from build123d import *

# Parameters (mm, degrees)
F0_R     = 3.048
F1_DEPTH = 6.35
F2_R     = 6.0325
F2_R_2   = 3.048
F3_DEPTH = 2.54
F5_DEPTH = 15.24
F6_R     = 1.397
F7_DEPTH = 9.525


with BuildPart() as f1:
    # F0 (on Top) → F1 (new body)
    with BuildSketch(Plane.XY):
        Circle(F0_R)
    extrude(amount=F1_DEPTH)

    # F2 (on face) → F3 (join)
    with BuildSketch(Plane(origin=(0, 0, 0), x_dir=(1, 0, 0), z_dir=(0, 0, -1))):
        Circle(F2_R)
        Circle(F2_R_2, mode=Mode.SUBTRACT)
        Circle(F2_R_2)
    extrude(amount=F3_DEPTH)

    # F4 (on face) → F5 (join)
    with BuildSketch(Plane(origin=(0, 0, -2.54), x_dir=(1, 0, 0), z_dir=(0, 0, -1))):
        Polygon((3.4925, -6.35), (-3.4925, 6.35), (-3.4925, -6.35), align=None)
        Polygon((3.4925, 6.35), (-3.4925, 6.35), (3.4925, -6.35), align=None)
    extrude(amount=F5_DEPTH)

    # F6 (on face) → F7 (join)
    with BuildSketch(Plane.XY.offset(6.35)):
        Circle(F6_R)
    extrude(amount=F7_DEPTH)


solid = f1.part
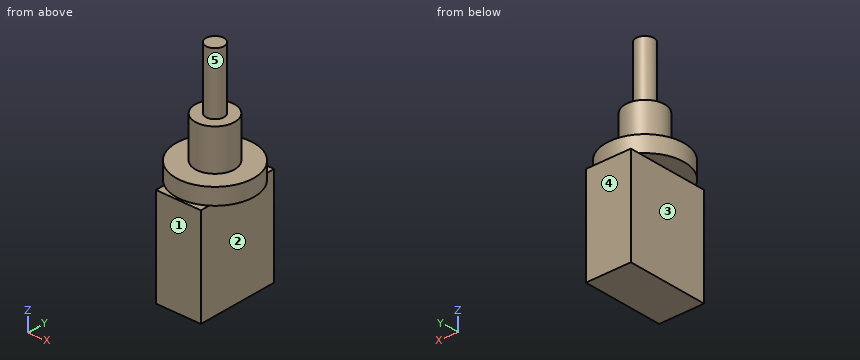
Geometry: final body of the model. Coordinates: model frame, mm. Face numbers are marked on the shaded views. A direction names the side the tool comes from. Round coordinates to 2 decimals unless told otherwise and drop trailing zeros. Loops run counter-clockwise (first coordinate to the right, second up) from the corner with the lowest first, then second, coordinate; pieces in that order, holes last. Notation, with made-up numbers: (-12.75, 27) - (-7.75, 27) arc R23 ccw to (-7.75, 56) - close; hole circle Ø11 at (31.5, -32). An arc over 180 degrees is marked (long way). Write each question's results on one line, items separated by ' | '. Start each with the question number.
1) Line query: probe 1 along X at (y, z) = (1.5, -12); probe 2 along Z at (x, y) = (0, 5.5); probe 3 along Z at (x, y) = (-1, 2.5). Output: solid intervals per line, ascending. Write a range as [from, to].
2) Cut plane C-C on z = 13.5. Return loops of the section in (x, y).
3) First-contact query: P1, Ø1.3, axis at x = 5.5, y = 0.5, coming from the -Z side; P2, Ø6, axis at x = -3, z = 9.5, coming from the +Y side; P3, Ø3, axis at x = 3.5, y = -2.5, coming from the +Z side. Flat tips, straight axial feed; report the tip coordinate or a pass-through.
4) Cut plane D-D on y = -3.75. Return loops of the section in (x, z).
5) Access query for the marked faces 1, 2, 3, 4 and 5. Directions: +Z, -Z, +X, -X, +Y, -Y. A direction counts if a zero-diameter tool reaches every point of the face in a straight line with its end or side. Return the directions, or none.
Verdict:
1) probe 1: x = [-3.49, 3.49] | probe 2: z = [-17.78, 0] | probe 3: z = [-17.78, 6.35]
2) outline: circle Ø2.79 at (0, 0)
3) P1: stops at z = -2.54 | P2: stops at y = 1.4 | P3: stops at z = 6.35
4) outline: (-4.73, -2.54) - (-3.49, -2.54) - (-3.49, -17.78) - (3.49, -17.78) - (3.49, -2.54) - (4.73, -2.54) - (4.73, 0) - (-4.73, 0) - close
5) face 1: +Z, -Z, +X, -X, -Y | face 2: -Z, +X, +Y, -Y | face 3: -Z, -X, +Y, -Y | face 4: +Z, -Z, +X, -X, +Y | face 5: +Z
